Part model, mm, in its own coordinate system. Face numbers are marked on the shaded views. Give positions to 0.01 mm unless a question says otherwise; leave off trailing zeros. Write each loop counter-clockwise with the first axis right and the second up, starting at its lowest first coordinate (ties: lowest second). Pieces come first, ordered by that corner, then holes. Notation, with made-up numbers: (-31.5, -25.75) - (24.5, -25.75) arc R26 ccw to (24.5, -0.75) - close; hole circle Ø4 at (-28.5, 26.25). An arc over 180 degrees is marked (long way). Answer in a Markdown table with one row per item. Add a question column.
1. Band-saw the part on A-A on x = -102.5. Write the cut outline in (y, z), plus the area to 3 significant figures.
2. Band-saw the part on B-B on x = -20.5. Write the cut outline in (y, z), plus the area to 3 significant figures.
3. Band-saw the part on C-C on x = -198. Write the cut outline in (y, z), plus the area to 3 significant figures.
4. Pull direction X, two halves, no side cores. Call the marked faces 1 and 2: released by +X, released by -X, zero draft, split by the parting line, or undercut.
5. Probe line 1 along X through (y, z) = (113.5, 10); line 2 along X through (y, z) = (-141, 18); line 3 along X through (y, z) = (42.5, 29). List the from-to ranges inside material, lowest first.
6. Drop flat-ended pins along their axis: pin 1 Ø6 at (x, y) = (155, 68.5) entering from +Z; pin 2 Ø5.5 at (y, z) = (136.73, 15) entering from +X; pin 3 Ø1.1 at (x, z) = (280.5, 15) entering from -Y; pin 4 Ø3.5 at (x, y) = (-289, -143.5) entering from +Z. Give the stop position or say it passes through.
```python
from build123d import *

# Parameters (mm, degrees)
F0_W      = 584
F0_H      = 350
F1_DEPTH  = 1
F2_W      = 1
F2_H      = 350
F3_DEPTH  = 30
F5_DEPTH  = 645
F6_W      = 1
F6_H      = 40
F7_DEPTH  = 30
F8_R      = 3
F9_DEPTH  = 565
F10_W     = 3
F10_H     = 250
F11_DEPTH = 28
F13_DEPTH = 291
F15_DEPTH = 25


with BuildPart() as f1:
    # F0 (on Top) → F1 (new body)
    with BuildSketch(Plane.XY):
        with Locations((0, -23.2696812643)):
            Rectangle(F0_W, F0_H)
    extrude(amount=F1_DEPTH)

    # F2 (on face) → F3 (join)
    with BuildSketch(Plane.XY.offset(1)):
        with Locations((-291.5, -23.2696812643)):
            Rectangle(F2_W, F2_H)
        with Locations((291.5, -23.2696812643)):
            Rectangle(F2_W, F2_H)
    extrude(amount=F3_DEPTH)

    # F4 (on face) → F5 (cut)
    with BuildSketch(Plane(origin=(-292, 0, 0), x_dir=(0, -1, 0), z_dir=(-1, 0, 0))):
        with BuildLine():
            Line((-136.7303187357, 15), (-136.7303187357, 10))
            ThreePointArc((-136.7303187357, 10), (-134.7165063478, 10.423477339), (-133.0438155245, 11.6221761335))
            ThreePointArc((-133.0438155245, 11.6221761335), (-132.0702481324, 13.1878901877), (-131.7303187357, 15))
            ThreePointArc((-131.7303187357, 15), (-132.1109210732, 16.9134171618), (-133.1947848298, 18.5355339059))
            Line((-133.1947848298, 18.5355339059), (-136.7303187357, 15))
        make_face()
        with BuildLine():
            Line((-151.7303187357, 10), (-136.7303187357, 10))
            ThreePointArc((-136.7303187357, 10), (-141.3497163983, 16.9134171618), (-133.1947848298, 18.5355339059))
            Line((-133.1947848298, 18.5355339059), (-120.7303187357, 31))
            Line((-120.7303187357, 31), (-151.7303187357, 31))
            Line((-151.7303187357, 31), (-151.7303187357, 10))
        make_face()
        with BuildLine():
            ThreePointArc((-133.1947848298, 18.5355339059), (-141.3497163983, 16.9134171618), (-136.7303187357, 10))
            Line((-136.7303187357, 10), (-136.7303187357, 15))
            Line((-136.7303187357, 15), (-133.1947848298, 18.5355339059))
        make_face()
        with BuildLine():
            ThreePointArc((-131.7303187357, 15), (-132.0702481324, 13.1878901877), (-133.0438155245, 11.6221761335))
            Line((-133.0438155245, 11.6221761335), (-113.6659916579, 31))
            Line((-113.6659916579, 31), (-120.7303187357, 31))
            Line((-120.7303187357, 31), (-133.1947848298, 18.5355339059))
            ThreePointArc((-133.1947848298, 18.5355339059), (-132.1109210732, 16.9134171618), (-131.7303187357, 15))
        make_face()
    extrude(amount=-F5_DEPTH, mode=Mode.SUBTRACT)

    # F6 (on face) → F7 (join)
    with BuildSketch(Plane.XY.offset(1)):
        with Locations((-280.5, 131.7303187357)):
            Rectangle(F6_W, F6_H)
        with Locations((280.5, 131.7303187357)):
            Rectangle(F6_W, F6_H)
    extrude(amount=F7_DEPTH)

    # F8 (on face) → F9 (cut)
    with BuildSketch(Plane(origin=(-281, 0, 0), x_dir=(0, -1, 0), z_dir=(-1, 0, 0))):
        with Locations((-136.7303187357, 15)):
            Circle(F8_R)
    extrude(amount=-F9_DEPTH, mode=Mode.SUBTRACT)

    # F10 (on face) → F11 (join)
    with BuildSketch(Plane.XY.offset(1)):
        with Locations((-288.5, -73.2696812643)):
            Rectangle(F10_W, F10_H)
        with Locations((288.5, -73.2696812643)):
            Rectangle(F10_W, F10_H)
    extrude(amount=F11_DEPTH)

    # F12 (on Right) → F13 (cut, symmetric)
    with BuildSketch(Plane.YZ):
        with BuildLine():
            ThreePointArc((-163.4468129313, 15.7271576906), (-160.4315110244, 20.4751748875), (-159.3769872614, 26))
            ThreePointArc((-159.3769872614, 26), (-165.262273131, 37.9131014568), (-178.2999187708, 40.4779352248))
            ThreePointArc((-178.2999187708, 40.4779352248), (-187.238776022, 18.2815552164), (-163.4468129313, 15.7271576906))
        make_face()
        with BuildLine():
            ThreePointArc((-178.2999187708, 40.4779352248), (-165.262273131, 37.9131014568), (-159.3769872614, 26))
            ThreePointArc((-159.3769872614, 26), (-160.4315110244, 20.4751748875), (-163.4468129313, 15.7271576906))
            Line((-163.4468129313, 15.7271576906), (-125.9341510427, 55.6401556402))
            Line((-125.9341510427, 55.6401556402), (-178.2999187708, 40.4779352248))
        make_face()
        with BuildLine():
            ThreePointArc((-112.4468129313, 15.7271576906), (-109.4315110244, 20.4751748875), (-108.3769872614, 26))
            ThreePointArc((-108.3769872614, 26), (-114.262273131, 37.9131014568), (-127.2999187708, 40.4779352248))
            ThreePointArc((-127.2999187708, 40.4779352248), (-136.238776022, 18.2815552164), (-112.4468129313, 15.7271576906))
        make_face()
        with BuildLine():
            ThreePointArc((-127.2999187708, 40.4779352248), (-114.262273131, 37.9131014568), (-108.3769872614, 26))
            ThreePointArc((-108.3769872614, 26), (-109.4315110244, 20.4751748875), (-112.4468129313, 15.7271576906))
            Line((-112.4468129313, 15.7271576906), (-74.9341510427, 55.6401556402))
            Line((-74.9341510427, 55.6401556402), (-127.2999187708, 40.4779352248))
        make_face()
        with BuildLine():
            ThreePointArc((-61.4468129313, 15.7271576906), (-58.4315110244, 20.4751748875), (-57.3769872614, 26))
            ThreePointArc((-57.3769872614, 26), (-63.262273131, 37.9131014568), (-76.2999187708, 40.4779352248))
            ThreePointArc((-76.2999187708, 40.4779352248), (-85.238776022, 18.2815552164), (-61.4468129313, 15.7271576906))
        make_face()
        with BuildLine():
            ThreePointArc((-76.2999187708, 40.4779352248), (-63.262273131, 37.9131014568), (-57.3769872614, 26))
            ThreePointArc((-57.3769872614, 26), (-58.4315110244, 20.4751748875), (-61.4468129313, 15.7271576906))
            Line((-61.4468129313, 15.7271576906), (-23.9341510427, 55.6401556402))
            Line((-23.9341510427, 55.6401556402), (-76.2999187708, 40.4779352248))
        make_face()
        with BuildLine():
            ThreePointArc((-10.4468129313, 15.7271576906), (-7.4315110244, 20.4751748875), (-6.3769872614, 26))
            ThreePointArc((-6.3769872614, 26), (-12.262273131, 37.9131014568), (-25.2999187708, 40.4779352248))
            ThreePointArc((-25.2999187708, 40.4779352248), (-34.238776022, 18.2815552164), (-10.4468129313, 15.7271576906))
        make_face()
        with BuildLine():
            ThreePointArc((-25.2999187708, 40.4779352248), (-12.262273131, 37.9131014568), (-6.3769872614, 26))
            ThreePointArc((-6.3769872614, 26), (-7.4315110244, 20.4751748875), (-10.4468129313, 15.7271576906))
            Line((-10.4468129313, 15.7271576906), (27.0658489573, 55.6401556402))
            Line((27.0658489573, 55.6401556402), (-25.2999187708, 40.4779352248))
        make_face()
        with BuildLine():
            ThreePointArc((40.5531870687, 15.7271576906), (43.5684889756, 20.4751748875), (44.6230127386, 26))
            ThreePointArc((44.6230127386, 26), (38.737726869, 37.9131014568), (25.7000812292, 40.4779352248))
            ThreePointArc((25.7000812292, 40.4779352248), (16.761223978, 18.2815552164), (40.5531870687, 15.7271576906))
        make_face()
        with BuildLine():
            ThreePointArc((25.7000812292, 40.4779352248), (38.737726869, 37.9131014568), (44.6230127386, 26))
            ThreePointArc((44.6230127386, 26), (43.5684889756, 20.4751748875), (40.5531870687, 15.7271576906))
            Line((40.5531870687, 15.7271576906), (78.0658489573, 55.6401556402))
            Line((78.0658489573, 55.6401556402), (25.7000812292, 40.4779352248))
        make_face()
    extrude(amount=F13_DEPTH, both=True, mode=Mode.SUBTRACT)

    # F14 (on face) → F15 (cut)
    with BuildSketch(Plane.XY.offset(1)):
        with BuildLine():
            ThreePointArc((-134.9042718153, 101.7303187357), (-144.5595998436, 94.3331327256), (-139.930476389, 83.0852468689))
            Line((-139.930476389, 83.0852468689), (-5.0262045737, 4.6525306972))
            ThreePointArc((-5.0262045737, 4.6525306972), (0, 3.297602564), (5.0262045737, 4.6525306972))
            Line((5.0262045737, 4.6525306972), (139.930476389, 83.0852468689))
            ThreePointArc((139.930476389, 83.0852468689), (144.5595998436, 94.3331327256), (134.9042718153, 101.7303187357))
            Line((134.9042718153, 101.7303187357), (-134.9042718153, 101.7303187357))
        make_face()
        with BuildLine():
            Line((-5.0262045737, -51.1918932258), (-139.930476389, -129.6246093974))
            ThreePointArc((-139.930476389, -129.6246093974), (-144.5595998436, -140.8724952541), (-134.9042718153, -148.2696812643))
            Line((-134.9042718153, -148.2696812643), (134.9042718153, -148.2696812643))
            ThreePointArc((134.9042718153, -148.2696812643), (144.5595998436, -140.8724952541), (139.930476389, -129.6246093974))
            Line((139.930476389, -129.6246093974), (5.0262045737, -51.1918932258))
            ThreePointArc((5.0262045737, -51.1918932258), (0, -49.8369650926), (-5.0262045737, -51.1918932258))
        make_face()
        with BuildLine():
            Line((-84.2441895854, -14.986847133), (-226.396906323, 81.1752847777))
            ThreePointArc((-226.396906323, 81.1752847777), (-236.6887665345, 81.7250871942), (-242, 72.8924506464))
            Line((-242, 72.8924506464), (-242, -119.431813175))
            ThreePointArc((-242, -119.431813175), (-236.6887665345, -128.2644497228), (-226.396906323, -127.7146473063))
            Line((-226.396906323, -127.7146473063), (-84.2441895854, -31.5525153956))
            ThreePointArc((-84.2441895854, -31.5525153956), (-79.8472832624, -23.2696812643), (-84.2441895854, -14.986847133))
        make_face()
        with BuildLine():
            Line((226.396906323, 81.1752847777), (84.2441895854, -14.986847133))
            ThreePointArc((84.2441895854, -14.986847133), (79.8472832624, -23.2696812643), (84.2441895854, -31.5525153956))
            Line((84.2441895854, -31.5525153956), (226.396906323, -127.7146473063))
            ThreePointArc((226.396906323, -127.7146473063), (236.6887665345, -128.2644497228), (242, -119.431813175))
            Line((242, -119.431813175), (242, 72.8924506464))
            ThreePointArc((242, 72.8924506464), (236.6887665345, 81.7250871942), (226.396906323, 81.1752847777))
        make_face()
    extrude(amount=-F15_DEPTH, mode=Mode.SUBTRACT)


solid = f1.part
```
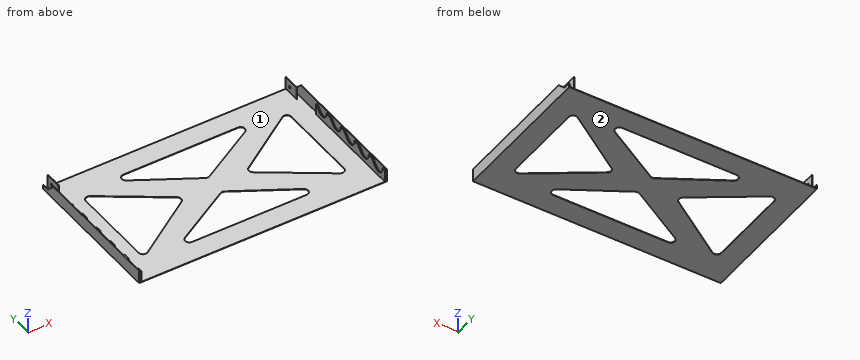
Values:
| question | item | result |
|---|---|---|
| 1 | outline | (-198.27, 0) - (-148.27, 0) - (-148.27, 1) - (-198.27, 1) - close; (-107.86, 0) - (-43.9, 0) - (-43.9, 1) - (-107.86, 1) - close; (-2.64, 0) - (61.32, 0) - (61.32, 1) - (-2.64, 1) - close; (101.73, 0) - (151.73, 0) - (151.73, 1) - (101.73, 1) - close |
| 1 | area | 228 mm² |
| 2 | outline | (-198.27, 0) - (-148.27, 0) - (-148.27, 1) - (-198.27, 1) - close; (-60.19, 0) - (13.65, 0) - (13.65, 1) - (-60.19, 1) - close; (101.73, 0) - (151.73, 0) - (151.73, 1) - (101.73, 1) - close |
| 2 | area | 174 mm² |
| 3 | outline | (-198.27, 0) - (-108.5, 0) - (-108.5, 1) - (-198.27, 1) - close; (61.97, 0) - (151.73, 0) - (151.73, 1) - (61.97, 1) - close |
| 3 | area | 180 mm² |
| 4 | face 1 | undercut |
| 4 | face 2 | zero draft |
| 5 | line 1 | x = -292 to -291, -281 to -280, 280 to 281, 291 to 292 |
| 5 | line 2 | x = -292 to -291, -290 to -287, 287 to 290, 291 to 292 |
| 5 | line 3 | x = -292 to -291, 291 to 292 |
| 6 | pin 1 | stops at z = 1 |
| 6 | pin 2 | passes through |
| 6 | pin 3 | stops at y = 111.73 |
| 6 | pin 4 | stops at z = 29 |
